Verification items for the finished model (mm, model axes). A direction names the side the tool comes from. Round coordinates to 2 decimals unless told otherwise and drop trailing zeros. Loops run counter-clockwise (first coordinate to the right, second up) from the corner with the lowest first, then second, coordinate; pieces in that order, holes last. Notation, with made-up numbers: (58.25, 22.5) -> (82.25, 22.5) arc R30 cw to (82.25, 50.5) -> close; hole circle Ø10 at (-13.75, -23). An arc over 180 degrees is marked (long way). Write item = value, one per line.
```python
from build123d import *

# Parameters (mm, degrees)
SKETCH1_R           = 4
SKETCH1_R_2         = 2.5
BOSS_EXTRUDE1_DEPTH = 1
SKETCH2_R           = 5
BOSS_EXTRUDE2_DEPTH = 30


with BuildPart() as part:
    # Sketch1 → Boss-Extrude1 (new body)
    with BuildSketch(Plane.XY):
        with BuildLine():
            Line((6.279627947, -6.447191082), (-136.991284981, -145.994478797))
            ThreePointArc((-136.991284981, -145.994478797), (-149.71810401, -145.826915663), (-149.550540875, -133.100096634))
            Line((-149.550540875, -133.100096634), (-6.279627947, 6.447191082))
            ThreePointArc((-6.279627947, 6.447191082), (6.447191082, 6.279627947), (6.279627947, -6.447191082))
        make_face()
        Circle(SKETCH1_R, mode=Mode.SUBTRACT)
        with Locations((-143.270912928, -139.547287716)):
            Circle(SKETCH1_R, mode=Mode.SUBTRACT)
        with Locations((-42.981273878, -41.864186315)):
            Circle(SKETCH1_R_2, mode=Mode.SUBTRACT)
        with Locations((-57.308365171, -55.818915086)):
            Circle(SKETCH1_R_2, mode=Mode.SUBTRACT)
    extrude(amount=BOSS_EXTRUDE1_DEPTH)

    # Sketch2 → Boss-Extrude2 (add)
    with BuildSketch(Plane.XY.offset(1)):
        with Locations((-100.28963905, -97.683101401)):
            Circle(SKETCH2_R)
    extrude(amount=BOSS_EXTRUDE2_DEPTH)


solid = part.part
```
(1) Material ranges on probe 1 along Y at (x, z) = (0, 0.2); probe 2 along Z at (x, y) = (-100.5, -87); probe 3 along X at (y, z) = (-94, 28), recorded low to high. Write a range as from..to.
Filled sheet:
probe_1 = -12.56..-4, 4..9
probe_2 = 0..1
probe_3 = -103.67..-96.91
(2) Sectioned sample at D-D, the plane z = 17.5. Record the cut outline in (x, y), and give its area (3 significant figures).
Filled sheet:
outline = circle Ø10 at (-100.29, -97.68)
area = 78.5 mm2
(3) Set-up check for faces 1 (the face through (-95.52, -96.18, 15.79)), 2 (the face through (-45.48, -41.75, 0.49)): record each of +Z, -Z, +X, -X, +Y, -Y from which the full face is reachable in a straight line by a thin tool's end or side.
Filled sheet:
face_1 = +Z
face_2 = +Z, -Z
(4) Draft check along X on faces 3 (the face through (-71, -75, 1)), 4 (the face through (-59.15, -54.13, 0.49)), 5 (the face through (-149.578, -145.967, 0.493)), 6 (the face through (-64.35, -75.24, 0.49)). Enter one of: released by +X, released by -X, zero draft, split by the parting line, or undercut.
Filled sheet:
face_3 = zero draft
face_4 = undercut
face_5 = split by the parting line
face_6 = released by +X
(5) Sectioned sample at C-C, the plane x = -69. Record the cut outline in (y, z), and give its area (3 significant figures).
Filled sheet:
outline = (-79.77, 0) -> (-54.64, 0) -> (-54.64, 1) -> (-79.77, 1) -> close
area = 25.1 mm2
(6) Sectioned sample at A-A, the plane y = 0. Record the cut outline in (x, z).
Filled sheet:
outline = (-12.9, 0) -> (-4, 0) -> (-4, 1) -> (-12.9, 1) -> close; (4, 0) -> (9, 0) -> (9, 1) -> (4, 1) -> close
(7) Go/stop test with a flat-tipped pin: pin 1 Ø13 at (x, y) = (-143.27, -139.55) entering from +Z. Record where the tip stops, or that it passes through.
Filled sheet:
pin_1 = 1
(8) Sectioned sample at B-B, the plane x = 0. Record the cut outline in (y, z), and give its area (3 significant figures).
Filled sheet:
outline = (-12.56, 0) -> (-4, 0) -> (-4, 1) -> (-12.56, 1) -> close; (4, 0) -> (9, 0) -> (9, 1) -> (4, 1) -> close
area = 13.6 mm2
